from build123d import *

# Parameters (mm, degrees)
SKETCH1_W           = 320
SKETCH1_H           = 200
SKETCH1_R           = 8.1
BOSS_EXTRUDE1_DEPTH = 30
SKETCH2_R           = 11
CUT_EXTRUDE1_DEPTH  = 20
SKETCH3_R           = 58.5
CUT_EXTRUDE2_DEPTH  = 5
CUT_EXTRUDE3_DEPTH  = 20
SKETCH5_R           = 2
CUT_EXTRUDE4_DEPTH  = 379.186461947
SKETCH6_R           = 40
CUT_EXTRUDE5_DEPTH  = 5
SKETCH7_R           = 30
CUT_EXTRUDE6_DEPTH  = 379.549864615
SKETCH8_R           = 2
CUT_EXTRUDE7_DEPTH  = 379.549864615
SKETCH9_R           = 1
CUT_EXTRUDE8_DEPTH  = 379.549864615


with BuildPart() as part:
    # Sketch1 → Boss-Extrude1 (new body)
    with BuildSketch(Plane.XY):
        with Locations((160, 100)):
            Rectangle(SKETCH1_W, SKETCH1_H)
        with Locations((25, 175)):
            Circle(SKETCH1_R, mode=Mode.SUBTRACT)
        with Locations((295, 175)):
            Circle(SKETCH1_R, mode=Mode.SUBTRACT)
        with Locations((25, 25)):
            Circle(SKETCH1_R, mode=Mode.SUBTRACT)
        with Locations((295, 25)):
            Circle(SKETCH1_R, mode=Mode.SUBTRACT)
    extrude(amount=BOSS_EXTRUDE1_DEPTH)

    # Sketch2 → Cut-Extrude1 (cut)
    with BuildSketch(Plane.XY.offset(30)):
        with Locations((295, 175)):
            Circle(SKETCH2_R)
        with Locations((25, 175)):
            Circle(SKETCH2_R)
        with Locations((25, 25)):
            Circle(SKETCH2_R)
        with Locations((295, 25)):
            Circle(SKETCH2_R)
    extrude(amount=-CUT_EXTRUDE1_DEPTH, mode=Mode.SUBTRACT)

    # Sketch3 → Cut-Extrude2 (cut)
    with BuildSketch(Plane(origin=(0, 0, 0), x_dir=(-1, 0, 0), z_dir=(0, 0, -1))):
        with Locations((-110, 100)):
            Circle(SKETCH3_R)
    extrude(amount=-CUT_EXTRUDE2_DEPTH, mode=Mode.SUBTRACT)

    # Sketch4 → Cut-Extrude3 (cut)
    with BuildSketch(Plane(origin=(0, 0, 5), x_dir=(-1, 0, 0), z_dir=(0, 0, -1))):
        with BuildLine():
            Line((-110, 116), (11.374075995, 116))
            Line((11.374075995, 116), (11.374075995, 84))
            Line((11.374075995, 84), (-110, 84))
            ThreePointArc((-110, 84), (-126, 100), (-110, 116))
        make_face()
    extrude(amount=-CUT_EXTRUDE3_DEPTH, mode=Mode.SUBTRACT)

    # Sketch5 → Cut-Extrude4 (cut, through all)
    with BuildSketch(Plane(origin=(0, 0, 25), x_dir=(-1, 0, 0), z_dir=(0, 0, -1))):
        with Locations((-110, 100)):
            Circle(SKETCH5_R)
    extrude(amount=-CUT_EXTRUDE4_DEPTH, mode=Mode.SUBTRACT)

    # Sketch6 → Cut-Extrude5 (cut)
    with BuildSketch(Plane(origin=(0, 0, 0), x_dir=(-1, 0, 0), z_dir=(0, 0, -1))):
        with Locations((-270, 100)):
            Circle(SKETCH6_R)
    extrude(amount=-CUT_EXTRUDE5_DEPTH, mode=Mode.SUBTRACT)

    # Sketch7 → Cut-Extrude6 (cut, through all)
    with BuildSketch(Plane(origin=(0, 0, 0), x_dir=(-1, 0, 0), z_dir=(0, 0, -1))):
        with Locations((-270, 100)):
            Circle(SKETCH7_R)
    extrude(amount=-CUT_EXTRUDE6_DEPTH, mode=Mode.SUBTRACT)

    # Sketch8 → Cut-Extrude7 (cut, through all)
    with BuildSketch(Plane(origin=(0, 0, 0), x_dir=(-1, 0, 0), z_dir=(0, 0, -1))):
        with Locations((-270, 135)):
            Circle(SKETCH8_R)
        with Locations((-235, 100)):
            Circle(SKETCH8_R)
        with Locations((-270, 65)):
            Circle(SKETCH8_R)
        with Locations((-305, 100)):
            Circle(SKETCH8_R)
    extrude(amount=-CUT_EXTRUDE7_DEPTH, mode=Mode.SUBTRACT)

    # Sketch9 → Cut-Extrude8 (cut, through all)
    with BuildSketch(Plane.XY.offset(30)):
        with Locations((110, 107.5)):
            Circle(SKETCH9_R)
        with Locations((117.5, 100)):
            Circle(SKETCH9_R)
        with Locations((110, 92.5)):
            Circle(SKETCH9_R)
        with Locations((102.5, 100)):
            Circle(SKETCH9_R)
    extrude(amount=-CUT_EXTRUDE8_DEPTH, mode=Mode.SUBTRACT)


solid = part.part
Input: part model. Units: mm. Frame: model coordinates. A direction names the side the tool comes from. Give positions to 0.01 mm unless a question says otherwise; leave off trailing zeros. Loops run counter-clockwise (first coordinate to the right, second up) from the corner with the lowest first, then second, coordinate; pieces in that order, holes last. Notation, with made-up numbers: (74.5, 63.25) - (124.5, 63.25) arc R19 ccw to (124.5, 92.25) - close; hole circle Ø1 at (-33.5, -15). An arc over 180 degrees is marked (long way). Use CSV: the item, a comma, the result in double quotes. Start each with the question number.
Item 1: Section D-D on x = 42. Return loops of the section in (y, z).
Item 2: Section C-C on z = 20. State how many separate pieces and enclosed holes the cut face has, then the cut area to 3 significant figures.
Item 3: Section A-A on y = 25. Return loops of the section in (x, z).
Item 4: Reachability of faces 5 (the cylindrical face through (29.4, 181.8, 4.9)), 6 (the flat face through (290.9, 167.7, 10)), 7 (the flat face through (56, 116, 15)) from +Z, -Z, +X, -X, +Y, -Y: full face, straight path, thin tool, end or side. Return the list, or none.
Item 5: Contact query for flat-ended pins moving along their axis: P1, Ø10, axis at x = 102.5, y = 138, coming from the -Z side; P2, Ø11, axis at x = 20.5, y = 25, coming from the +Z side. Output: stop coordinate, or through.
Item 6: Section B-B on x = 295. Return loops of the section in (y, z), then the cut area to 3 significant figures.
Item 7: Line query: line 1 (Y direction, x = 270, z = 17.5); line 2 (Y direction, x = 25, z = 24); line 3 (X direction, y = 25, z = 7.5). Output: solid intervals per line, ascending.
Item 8: Mould query, pull axis Y, two halves, no side actions, for faces 1 (the flat face through (320, 99, 15)), 2 (the cylindrical face through (126, 100, 15)), 3 (the flat face through (158, 200, 15)), 4 (the cylindrical face through (83.01, 48.1, 2.46)). Classes: pulls with the +Y half, pulls with the -Y half, needs draft (parallel to the pull), parting line crosses it, or undercut.
Ans:
1,outline,"(0, 0) - (200, 0) - (200, 30) - (0, 30) - close; hole (84, 5) - (116, 5) - (116, 25) - (84, 25) - close"
2,separate pieces,"1"
2,enclosed holes,"9"
2,area,"55,700 mm2"
3,outline,"(0, 0) - (16.9, 0) - (16.9, 10) - (14, 10) - (14, 30) - (0, 30) - close; (33.1, 0) - (286.9, 0) - (286.9, 10) - (284, 10) - (284, 30) - (36, 30) - (36, 10) - (33.1, 10) - close; (303.1, 0) - (320, 0) - (320, 30) - (306, 30) - (306, 10) - (303.1, 10) - close"
4,face 5,"+Z, -Z"
4,face 6,"+Z"
4,face 7,"-X"
5,P1,"stops at z = 5"
5,P2,"stops at z = 10"
6,outline,"(0, 0) - (16.9, 0) - (16.9, 10) - (14, 10) - (14, 30) - (0, 30) - close; (33.1, 0) - (68.78, 0) - (68.78, 5) - (83.42, 5) - (83.42, 30) - (36, 30) - (36, 10) - (33.1, 10) - close; (116.58, 5) - (131.22, 5) - (131.22, 0) - (166.9, 0) - (166.9, 10) - (164, 10) - (164, 30) - (116.58, 30) - close; (183.1, 0) - (200, 0) - (200, 30) - (186, 30) - (186, 10) - (183.1, 10) - close"
6,area,"3,650 mm2"
7,line 1,"y = 0 to 63, 67 to 70, 130 to 133, 137 to 200"
7,line 2,"y = 0 to 14, 36 to 84, 116 to 164, 186 to 200"
7,line 3,"x = 0 to 16.9, 33.1 to 286.9, 303.1 to 320"
8,face 1,"needs draft"
8,face 2,"undercut"
8,face 3,"pulls with the +Y half"
8,face 4,"undercut"
